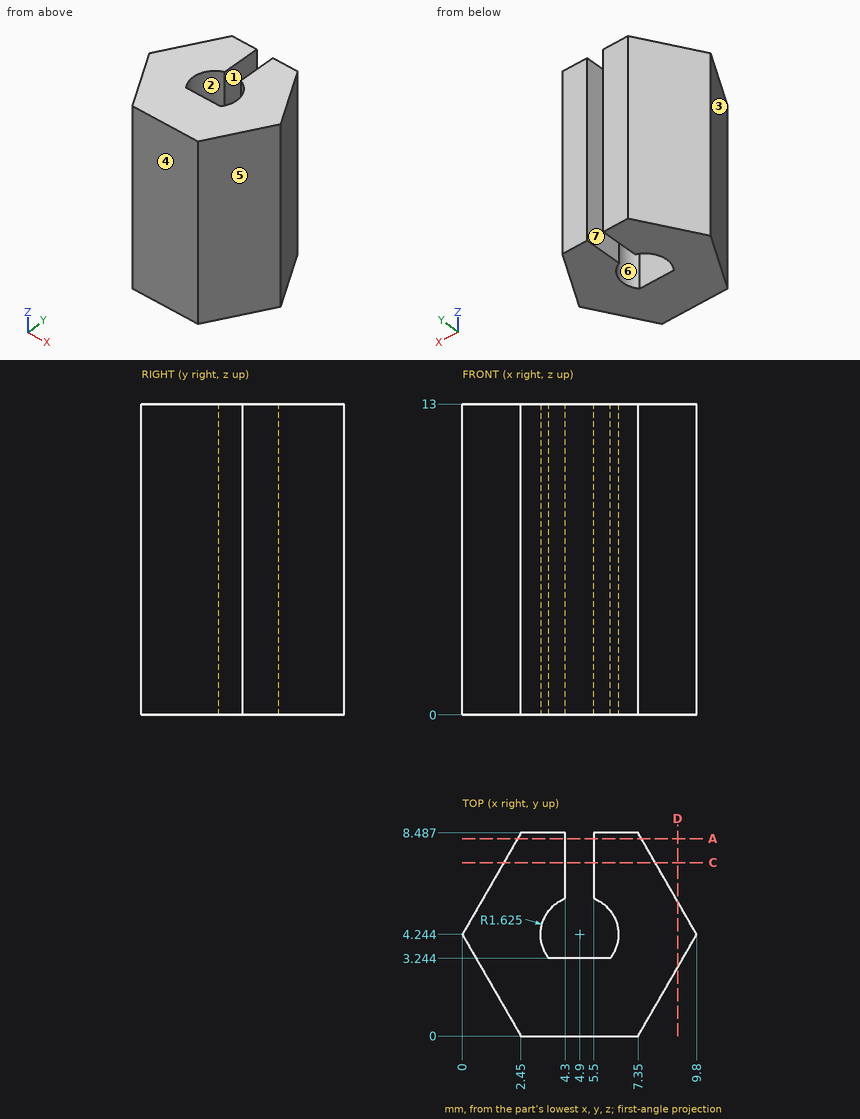
Answer from the drawing. Dimensions are ordinates in mm from the lowest x, y and z of the part. A direction names the side the tool comes from. Give positions to 0.01 mm unless a question says otherwise; leave off trailing zeros. Loops run counter-clockwise (first coordinate to the right, second up) from the corner with the lowest first, then second, coordinate; pieces in that order, holes last. Notation, with made-up numbers: (-30, 12) - (-18, 12) arc R34 cw to (-18, 48) - close; hole circle Ø7 at (-17.5, -10.75). An arc over 180 degrees is marked (long way). Write each question's results on one line, items separated by ' | '.
1. Flat-ended cylindrical pins translate along their axes: P1, Ø1.5, axis at x = 8, z = 8.5, coming from the -Y side; P2, Ø3, axis at y = 6, z = 5.5, coming from the +X side; P3, Ø2, axis at y = 4.5, z = 5, coming from the +X side; P4, Ø1.4, axis at y = 7.5, z = 4, coming from the -X side (1 decimal). Find the tip coordinate at first contact, or state that the pin passes through.
Resolved:
P1: stops at y = 0 | P2: stops at x = 9.65 | P3: stops at x = 9.8 | P4: stops at x = 1.5
2. Which of the six approach directions +Z, -Z, +X, -X, +Y, -Y give full straight-line access (tool end or side, diameter ignored) to the marked faces 1, 2 and 3?
Resolved:
face 1: +Z, -Z, +Y | face 2: +Z, -Z | face 3: +Z, -Z, -X, -Y
3. For a pull along X with two mould halves and no side action, classify the marked faces 4, 5, 6 and 7 as +X half, -X half, draft (parallel to the pull), parting line (faces both ways), or undercut.
Resolved:
face 4: draft | face 5: +X half | face 6: undercut | face 7: undercut
4. Find section C-C, the plane y = 7.25. Write down the section's boundary in (x, z) (1 decimal).
Resolved:
outline: (1.7, 0) - (4.3, 0) - (4.3, 13) - (1.7, 13) - close; (5.5, 0) - (8.1, 0) - (8.1, 13) - (5.5, 13) - close
5. Find section D-D, the plane x = 9. Write down the section's boundary in (y, z).
Resolved:
outline: (2.86, 0) - (5.63, 0) - (5.63, 13) - (2.86, 13) - close
6. Find section A-A, the plane y = 8.25. Write down the section's boundary in (x, z).
Resolved:
outline: (2.31, 0) - (4.3, 0) - (4.3, 13) - (2.31, 13) - close; (5.5, 0) - (7.49, 0) - (7.49, 13) - (5.5, 13) - close
7. Consider probe 1 along X at (y, z) = (5, 6) (1 decimal); probe 2 along X at (y, z) = (7.25, 11.5) (1 decimal); probe 3 along Y at (x, z) = (5.75, 4) (1 decimal). Determine where each line is inside the solid, lowest interval first. Write a range as from..to.
Resolved:
probe 1: x = 0.4..3.5, 6.3..9.4 | probe 2: x = 1.7..4.3, 5.5..8.1 | probe 3: y = 0..3.2, 5.6..8.5
